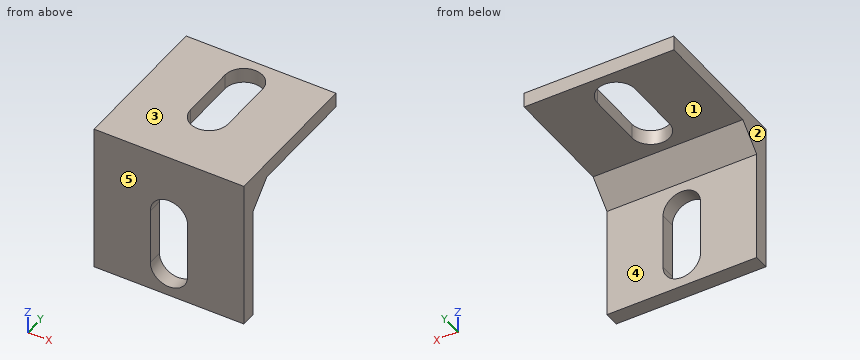
from build123d import *

# Parameters (mm, degrees)
BODY_DEPTH          = 10
FIXATION_HOLE_DEPTH = 29.705400189


with BuildPart() as part:
    # Sketch1 → Body (new, symmetric)
    with BuildSketch(Plane(origin=(0, 0, 0), x_dir=(0, 0, -1), z_dir=(1, 0, 0))):
        Polygon((20, 0), (0, 0), (0, 20), (2, 20), (2, 5), (5, 2), (20, 2), align=None)
    extrude(amount=BODY_DEPTH, both=True)

    # Sketch3 → Fixation_Hole (cut, through all)
    with BuildSketch(Plane(origin=(0, 0, -2), x_dir=(-1, 0, 0), z_dir=(0, 0, -1))):
        with BuildLine():
            Line((-2.5, 8.75), (-2.5, 16.25))
            ThreePointArc((-2.5, 16.25), (0, 18.75), (2.5, 16.25))
            Line((2.5, 16.25), (2.5, 8.75))
            ThreePointArc((2.5, 8.75), (0, 6.25), (-2.5, 8.75))
        make_face()
    fixation_hole = extrude(amount=-FIXATION_HOLE_DEPTH, mode=Mode.SUBTRACT)

    # Mirror1: Fixation_Hole across plane
    add(fixation_hole.mirror(Plane(origin=(0, 0, 0), x_dir=(0, -0.7071067811865476, 0.7071067811865475), z_dir=(0, -0.7071067811865475, -0.7071067811865476))), mode=Mode.SUBTRACT)


solid = part.part
Here's how the part is built. I have some questions about the finished solid (model axes, mm). Face numbers are marked on the shaded views. A direction names the side the tool comes from. Give positions to 0.01 mm unless a question says otherwise; leave off trailing zeros. Order: outer loops, then holes, each group sorted by start corner. A loop starts at its lowest first (then second) coordinate and runs counter-clockwise, first axis right, second up. Notation, with made-up numbers: (12.25, 76.5) -> (37.25, 76.5) arc R25 ccw to (37.25, 105.5) -> close; hole circle Ø3 at (62.5, 52.5). An arc over 180 degrees is marked (long way). One line per item, written item: value. Start each with the question number.
1. I need wall thicknesses on probe 1 along Z at (x, y) = (4, 7); probe 2 along Y at (x, z) = (9, -10.25); probe 3 along X at (y, z) = (1, -6.75). Which ranges of each line are inside material? Lowest first, please. Write a range as from..to.
2. Will these pins go through, and if not, where does the flat tip stop? pin 1 Ø5 at (x, y) = (-4, 7) entering from +Z; pin 2 Ø4.5 at (x, y) = (-1.5, 16) entering from -Z; pin 3 Ø1.5 at (x, y) = (-3.5, 3) entering from -Z; pin 4 Ø3 at (x, z) = (-1.5, -17.5) entering from +Y.
3. We'd pull the mould along Z, two halves only. Please class the marked faces 1, 2 and 3: released by +Z, released by -Z, zero draft, split by the parting line, or undercut.
4. Imagine slicing it at B-B, the plane z = -12.5. List the corners of the cut face in (x, y) for me.
5. Imagine slicing it at A-A, the plane x = -2. List the corners of the cut face in (y, z) for me, plus the area to 3 significant figures.
6. Imagine slicing it at D-D, the plane y = 8.25. List the corners of the cut face in (x, z) for me.
7. Imagine slicing it at C-C, the plane x = 0. List the corners of the cut face in (y, z) for me.
8. For the marked faces 4 and 5, which set-ups out of +Z, -Z, +X, -X, +Y, -Y let a thin tool reach every point of the face, with its end or its side?
Values follow:
1. probe 1: z = -2..0
1. probe 2: y = 0..2
1. probe 3: x = -10..-1.5, 1.5..10
2. pin 1: stops at z = 0
2. pin 2: stops at z = -2
2. pin 3: stops at z = -4.75
2. pin 4: stops at y = 2
3. face 1: released by -Z
3. face 2: zero draft
3. face 3: released by +Z
4. outline: (-10, 0) -> (-2.5, 0) -> (-2.5, 2) -> (-10, 2) -> close; (2.5, 0) -> (10, 0) -> (10, 2) -> (2.5, 2) -> close
5. outline: (0, -20) -> (2, -20) -> (2, -17.75) -> (0, -17.75) -> close; (0, -7.25) -> (2, -7.25) -> (2, -5) -> (5, -2) -> (7.25, -2) -> (7.25, 0) -> (0, 0) -> close; (17.75, -2) -> (20, -2) -> (20, 0) -> (17.75, 0) -> close
5. area: 38.5 mm2
6. outline: (-10, -2) -> (-2.45, -2) -> (-2.45, 0) -> (-10, 0) -> close; (2.45, -2) -> (10, -2) -> (10, 0) -> (2.45, 0) -> close
7. outline: (0, -20) -> (2, -20) -> (2, -18.75) -> (0, -18.75) -> close; (0, -6.25) -> (2, -6.25) -> (2, -5) -> (5, -2) -> (6.25, -2) -> (6.25, 0) -> (0, 0) -> close; (18.75, -2) -> (20, -2) -> (20, 0) -> (18.75, 0) -> close
8. face 4: -Z, +X, -X, +Y
8. face 5: +Z, -Z, +X, -X, -Y
